Geometry: see drawing. Coordinates: mm, zero at the bounding-box minimum. Coordinates: 2 decimals unless noted, no trailing zeros. Loops run counter-clockwise (first coordinate to the right, second up) from the corner with the lowest first, then second, coordinate; pieces in that order, holes last. Notation, with made-up numbers: (32.25, 8.25) - (87.25, 8.25) arc R30 cw to (87.25, 45.25) - close; hole circle Ø1 at (2.25, 74). An arc over 180 degrees is marked (long way). Write each question's results on one line, items separated by ' | '. Start each with the question number.
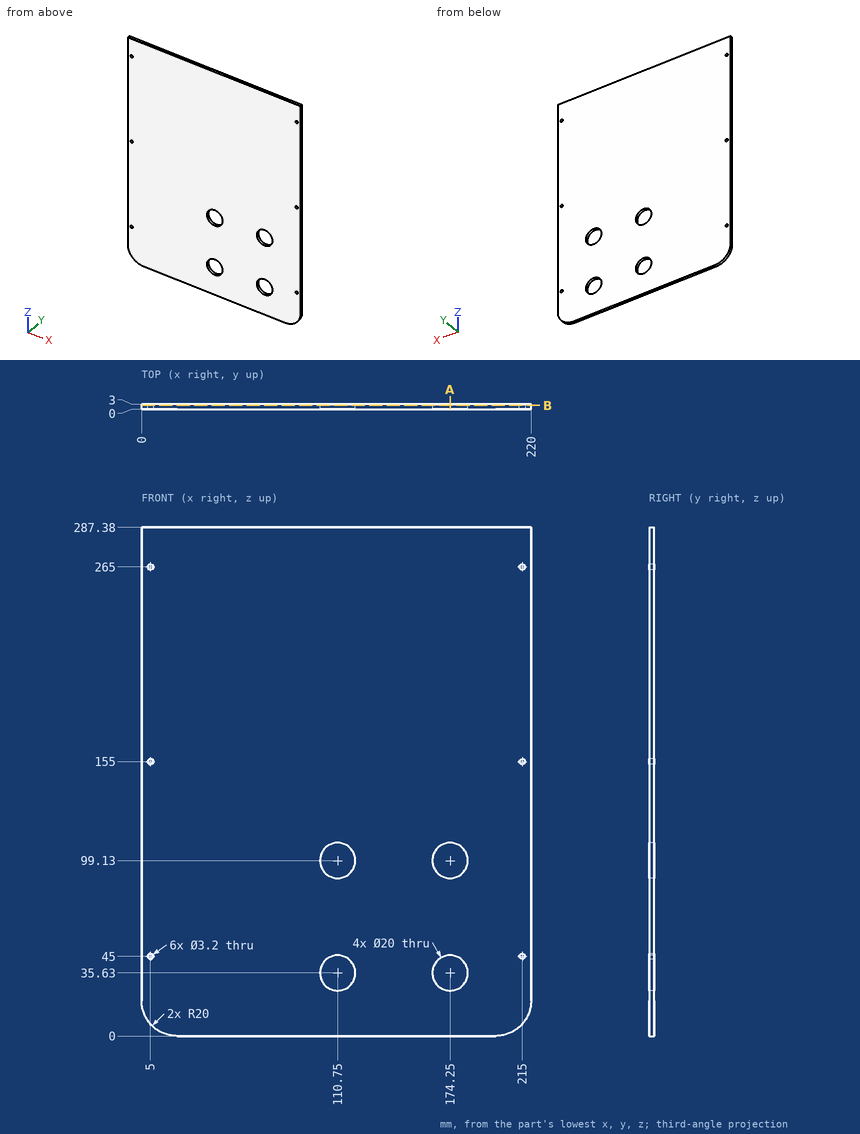
1) Material intervals for line 1 (X direction, y = 1.3, z = 155); line 2 (Z direction, x = 110.75, y = 1.4); line 3 (Z direction, x = 215, y = 0.8), sorted ascending. Write a range as [from, to].
2) Section query A-A on x = 174.25. Output: boundary loops of the cut face in (y, z).
3) Section query B-B on y = 2.2. Count the separate pieces of the cut face and the enclosed holes in it, and give its area (3 significant figures).
Returned:
1) line 1: x = [0, 3.4], [6.6, 213.4], [216.6, 220] | line 2: z = [0, 25.63], [45.63, 89.13], [109.13, 287.38] | line 3: z = [6.77, 43.4], [46.6, 153.4], [156.6, 263.4], [266.6, 287.38]
2) outline: (0, 0) - (3, 0) - (3, 25.63) - (0, 25.63) - close; (0, 45.63) - (3, 45.63) - (3, 89.13) - (0, 89.13) - close; (0, 109.13) - (3, 109.13) - (3, 287.38) - (0, 287.38) - close
3) separate pieces: 1 | enclosed holes: 10 | area: 61,700 mm²
